from build123d import *

# Parameters (mm, degrees)
F1_DEPTH = 56.388
F2_W     = 13.5290427133
F2_H     = 11.8184806779
F3_DEPTH = 16.51


with BuildPart() as f1:
    # F0 (on Front) → F1 (new body)
    with BuildSketch(Plane.XZ):
        Polygon((0, 38.2545590401), (0, 0), (59.4034036621, 0), (59.4034036621, 38.2545590401), (45.8743609488, 38.2545590401), (45.8743609488, 16.7946852744), (13.5290427133, 16.7946852744), (13.5290427133, 38.2545590401), align=None)
    extrude(amount=-F1_DEPTH)

    # F2 (on face) → F3 (cut)
    with BuildSketch(Plane.XY.offset(38.2545590401)):
        with Locations((52.6388823055, 16.6865340434)):
            Rectangle(F2_W, F2_H)
    extrude(amount=-F3_DEPTH, mode=Mode.SUBTRACT)


solid = f1.part
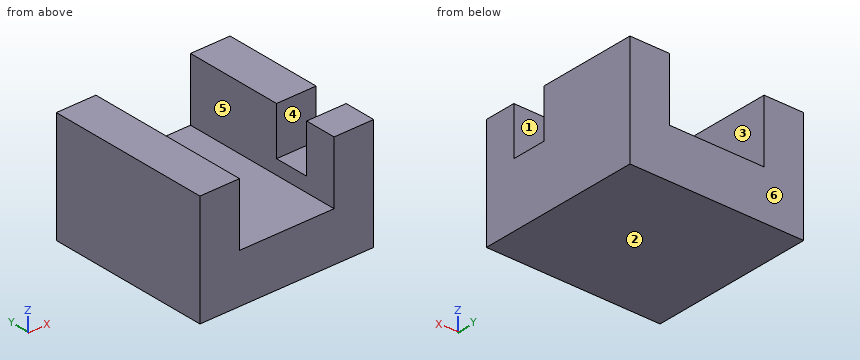
Work out the finished part from the listing and answer in its coordinate system (mm). Face numbers are marked on the shaded views. A direction names the side the tool comes from. Coordinates: 2 decimals unless noted, no trailing zeros. Write each loop counter-clockwise with the first axis right and the second up, starting at its lowest first coordinate (ties: lowest second). Pieces come first, ordered by that corner, then holes. Notation, with made-up numbers: M 33,-28 L 37,-28 A24 cw 37,-8 Z; hole C 30,87.25 d7. An arc over 180 degrees is marked long. Write item = value, one per line.
1. A flat-ended cylindrical pin translates along its axis: pin 1 (3.5 mm diameter, centred on x = 52.5, y = 14, fed in from +Z). Find the tip coordinate at first contact, or state that the pin passes through.
Solution:
pin_1 = 21.74
2. Determine the mould class of the marked faces 4, 5 and 6 for opening direction Y: released by +Y, released by -Y, zero draft, split by the parting line, or undercut.
Solution:
face_4 = undercut
face_5 = zero draft
face_6 = released by +Y
3. Straight lines are drawn through the part: line 1 (Y direction, x = 49, z = 32); line 2 (X direction, y = 52, z = 25.5); line 3 (Z direction, x = 19, y = 16.5). For each, find the intervals that lie inside material, in ascending order. Write a range as from..to.
Solution:
line_1 = 0..10.78, 22.6..56.39
line_2 = 0..13.53, 45.87..59.4
line_3 = 0..16.79
4. The part is cut by section A-A (z = 26). Determine the outline of the cut face in (x, y).
Solution:
outline = M 0,0 L 13.53,0 L 13.53,56.39 L 0,56.39 Z; M 45.87,0 L 59.4,0 L 59.4,10.78 L 45.87,10.78 Z; M 45.87,22.6 L 59.4,22.6 L 59.4,56.39 L 45.87,56.39 Z
5. The part is cut by section B-B (x = 55.5). Determine the outline of the cut face in (y, z).
Solution:
outline = M 0,0 L 56.39,0 L 56.39,38.25 L 22.6,38.25 L 22.6,21.74 L 10.78,21.74 L 10.78,38.25 L 0,38.25 Z
6. The part is cut by section D-D (x = 28). Determine the outline of the cut face in (y, z), then the cut area to 3 significant figures.
Solution:
outline = M 0,0 L 56.39,0 L 56.39,16.79 L 0,16.79 Z
area = 947 mm2
7. For the marked faces 1, 2 and 3, determine the directions among +Z, -Z, +X, -X, +Y, -Y from which every point of the face is accessible in a straight line to the end or side of a thin tool.
Solution:
face_1 = +Z, +X
face_2 = -Z, +X, -X, +Y, -Y
face_3 = +Z, +Y, -Y
8. The part is cut by section C-C (y = 19.5). Determine the outline of the cut face in (x, z), then the cut area to 3 significant figures.
Solution:
outline = M 0,0 L 59.4,0 L 59.4,21.74 L 45.87,21.74 L 45.87,16.79 L 13.53,16.79 L 13.53,38.25 L 0,38.25 Z
area = 1,350 mm2
